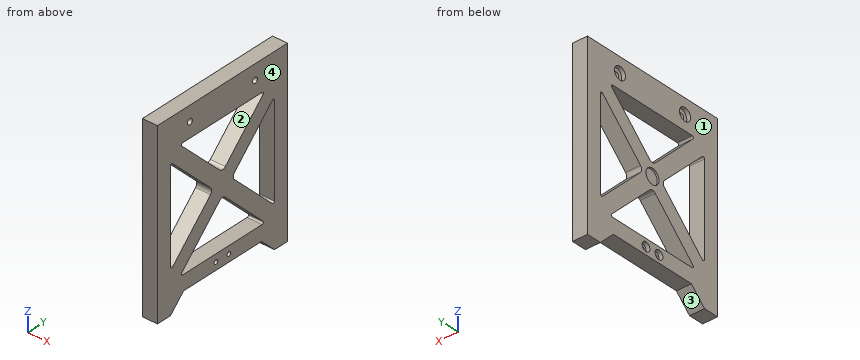
```python
from build123d import *

# Parameters (mm, degrees)
F1_DEPTH       = 10
F2_R           = 1
F3_D           = 3.8
F3_CBORE_D     = 8.5
F3_CBORE_DEPTH = 2.5
F4_R           = 5
F5_DEPTH       = 1.2
F8_D           = 2.8
F8_CBORE_D     = 6
F8_CBORE_DEPTH = 2.5


with BuildPart() as f1:
    # F0 (on Right) → F1 (new body)
    with BuildSketch(Plane.YZ):
        Polygon((40.0512183458, -60), (50, -60), (50, 60), (-50, 60), (-50, -60), (-40, -60), (-29.9487816542, -50), (30.0512183458, -50), align=None)
        with BuildLine():
            Line((2.1213203436, -9.1923881554), (32.9289321881, -40))
            Line((32.9289321881, -40), (-32.9289321881, -40))
            Line((-32.9289321881, -40), (-2.1213203436, -9.1923881554))
            ThreePointArc((-2.1213203436, -9.1923881554), (0, -8.313708499), (2.1213203436, -9.1923881554))
        make_face(mode=Mode.SUBTRACT)
        with BuildLine():
            Line((-9.1923881554, -2.1213203436), (-40, -32.9289321881))
            Line((-40, -32.9289321881), (-40, 32.9289321881))
            Line((-40, 32.9289321881), (-9.1923881554, 2.1213203436))
            ThreePointArc((-9.1923881554, 2.1213203436), (-8.313708499, 0), (-9.1923881554, -2.1213203436))
        make_face(mode=Mode.SUBTRACT)
        with BuildLine():
            Line((40, 32.9289321881), (40, -32.9289321881))
            Line((40, -32.9289321881), (9.1923881554, -2.1213203436))
            ThreePointArc((9.1923881554, -2.1213203436), (8.313708499, 0), (9.1923881554, 2.1213203436))
            Line((9.1923881554, 2.1213203436), (40, 32.9289321881))
        make_face(mode=Mode.SUBTRACT)
        with BuildLine():
            Line((-32.9289321881, 40), (32.9289321881, 40))
            Line((32.9289321881, 40), (2.1213203436, 9.1923881554))
            ThreePointArc((2.1213203436, 9.1923881554), (0, 8.313708499), (-2.1213203436, 9.1923881554))
            Line((-2.1213203436, 9.1923881554), (-32.9289321881, 40))
        make_face(mode=Mode.SUBTRACT)
    extrude(amount=F1_DEPTH)

    # F2
    f2_edges = [f1.edges().sort_by_distance(p)[0] for p in [
        (5, -32.928932, 40),
        (5, 32.928932, 40),
        (5, -40, 32.928932),
        (5, -40, -32.928932),
        (5, -32.928932, -40),
        (5, 40, 32.928932),
        (5, 40, -32.928932),
        (5, 32.928932, -40),
    ]]
    fillet(f2_edges, radius=F2_R)

    # F3 (through all)
    with Locations(Plane(origin=(0, 0, 0), x_dir=(0, 1, 0), z_dir=(-1, 0, 0))):
        with Locations((-25, -50), (25, -50)):
            CounterBoreHole(F3_D / 2, F3_CBORE_D / 2, F3_CBORE_DEPTH)

    # F4 (on face) → F5 (cut)
    with BuildSketch(Plane(origin=(0, 0, 0), x_dir=(0, -1, 0), z_dir=(-1, 0, 0))):
        Circle(F4_R)
    extrude(amount=-F5_DEPTH, mode=Mode.SUBTRACT)

    # F8 (through all)
    with Locations(Plane(origin=(0, 0, 0), x_dir=(0, -1, 0), z_dir=(-1, 0, 0))):
        with Locations((-5, -45), (5, -45)):
            CounterBoreHole(F8_D / 2, F8_CBORE_D / 2, F8_CBORE_DEPTH)


solid = f1.part
```
Part model, mm, in its own coordinate system. Face numbers are marked on the shaded views. A direction names the side the tool comes from. Round coordinates to 2 decimals unless told otherwise and drop trailing zeros. Loops run counter-clockwise (first coordinate to the right, second up) from the corner with the lowest first, then second, coordinate; pieces in that order, holes last.
1. Flat gauge pins, fed straight in: pin 1 (5 mm diameter, centred on x = 5.5, y = 15, fed in from -Z); pin 2 (7 mm diameter, centred on y = -25, z = 50, fed in from -X); pin 3 (1.7 mm diameter, centred on y = -5, z = -45, fed in from +X). Where does each tip first touch, or does it go through?
Solutions:
pin 1: stops at z = -50
pin 2: stops at x = 2.5
pin 3: passes through
2. 3-axis set-ups, long thin cutter, end or side, ignore diameter. For the marked faces 1 and 2: which of +Z, -Z, +X, -X, +Y, -Y reach the whole face in a straight line?
Solutions:
face 1: +Z, -Z, -X, +Y, -Y
face 2: +X, -X
3. Slice it at B-B (y = 12.5). Give the cut face in (x, z), and give its area (3 significant figures).
Solutions:
outline: (0, -50) - (10, -50) - (10, -40) - (0, -40) - close; (0, -19.57) - (10, -19.57) - (10, -5.43) - (0, -5.43) - close; (0, 5.43) - (10, 5.43) - (10, 19.57) - (0, 19.57) - close; (0, 40) - (10, 40) - (10, 60) - (0, 60) - close
area: 583 mm2
4. Slice it at C-C (y = -25). Give the cut face in (x, z), and give its area (3 significant figures).
Solutions:
outline: (0, -50) - (10, -50) - (10, -40) - (0, -40) - close; (0, -32.07) - (10, -32.07) - (10, -17.93) - (0, -17.93) - close; (0, 17.93) - (10, 17.93) - (10, 32.07) - (0, 32.07) - close; (0, 40) - (10, 40) - (10, 48.1) - (2.5, 48.1) - (2.5, 45.75) - (0, 45.75) - close; (0, 54.25) - (2.5, 54.25) - (2.5, 51.9) - (10, 51.9) - (10, 60) - (0, 60) - close
area: 533 mm2
5. Drill centre lines: line 1 along Z through (x, y) = (0.25, 0); line 2 along Y through (x, z) = (1.7, 50); line 3 along Z through (x, y) = (4.25, -5). Where is each one in solid material? Low to high.
Solutions:
line 1: z = -50 to -40, -8.31 to -5, 5 to 8.31, 40 to 60
line 2: y = -50 to -29.25, -20.75 to 20.75, 29.25 to 50
line 3: z = -50 to -46.4, -43.6 to -40, -12.07 to 12.07, 40 to 60
6. Two-plate mould, pull along Y, no slides. Class the marked faces 3 and 4: pulls with the +Y half, pulls with the -Y half, needs draft (parallel to the pull), parting line crosses it, or undercut.
Solutions:
face 3: undercut
face 4: needs draft
7. Slice it at A-A (z = 0). Give the cut face in (x, y).
Solutions:
outline: (0, -50) - (10, -50) - (10, -40) - (0, -40) - close; (0, -8.31) - (10, -8.31) - (10, 8.31) - (0, 8.31) - (0, 5) - (1.2, 5) - (1.2, -5) - (0, -5) - close; (0, 40) - (10, 40) - (10, 50) - (0, 50) - close
8. Slice it at D-D (z = -45). Give the cut face in (x, y), and give its area (3 significant figures).
Solutions:
outline: (0, -50) - (10, -50) - (10, -6.4) - (2.5, -6.4) - (2.5, -8) - (0, -8) - close; (0, -2) - (2.5, -2) - (2.5, -3.6) - (10, -3.6) - (10, 3.6) - (2.5, 3.6) - (2.5, 2) - (0, 2) - close; (0, 8) - (2.5, 8) - (2.5, 6.4) - (10, 6.4) - (10, 50) - (0, 50) - close
area: 928 mm2
